Here's the drawing with two shaded views (mm, measured from the low corner). I have some questions. Round coordinates to 2 decimals unless told otherwise and drop trailing zeros. Order: outer loops, then holes, each group sorted by start corner. A loop starts at its lowest first (then second) coordinate and runs counter-clockwise, first axis right, second up.
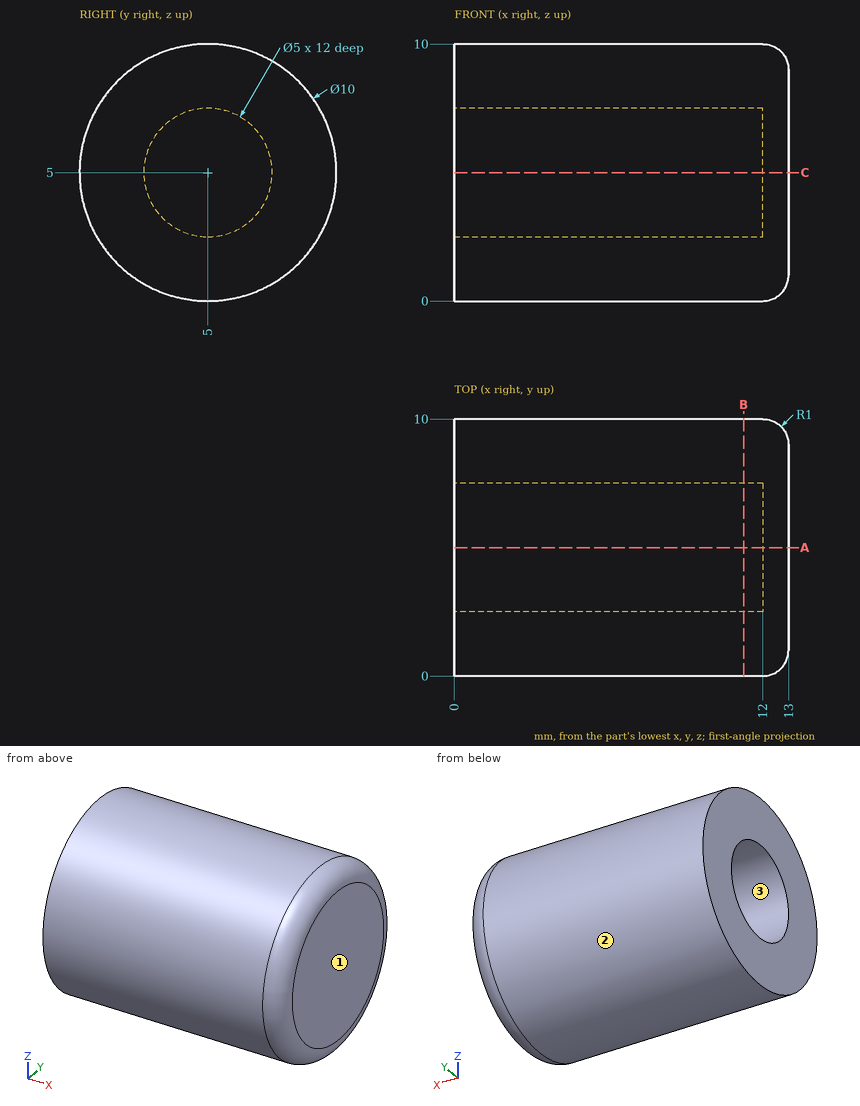
1. If we section it at B-B, the plane x = 11.25: Write out the boundary of the cut face in (y, z), and give its area (3 significant figures).
Evaluation:
outline: circle Ø10 at (5, 5); hole circle Ø5 at (5, 5)
area: 58.9 mm2
2. I'm going to push flat-ended pins straight in: P1, Ø4, axis at y = 5, z = 5, coming from the -X side; P2, Ø3, axis at x = 8.5, y = 8.5, coming from the -Z side; P3, Ø4, axis at x = 11, y = 8, coming from the +Z side. Where does each tip first touch, or does it pass through?
Evaluation:
P1: stops at x = 12
P2: stops at z = 0.42
P3: stops at z = 9.9
3. I need wall thicknesses on probe 1 along Y at (x, z) = (7, 5); probe 2 along X at (y, z) = (5.5, 5.5); probe 3 along Z at (x, y) = (11.75, 4.75). Which ranges of each line are inside material? Lowest first, please.
Evaluation:
probe 1: y = 0 to 2.5, 7.5 to 10
probe 2: x = 12 to 13
probe 3: z = 0.01 to 2.51, 7.49 to 9.99
4. If we mould it in two halves opening along Y, with no side actions, what happens to the marked faces 1, 2 and 3? For each: released by +Y, released by -Y, zero draft, split by the parting line, or undercut.
Evaluation:
face 1: zero draft
face 2: split by the parting line
face 3: undercut
5. If we section it at A-A, the plane y = 5: Write out the boundary of the cut face in (x, z).
Evaluation:
outline: (0, 0) - (12, 0) arc R1 ccw to (13, 1) - (13, 9) arc R1 ccw to (12, 10) - (0, 10) - (0, 7.5) - (12, 7.5) - (12, 2.5) - (0, 2.5) - close
